```python
from build123d import *

# Parameters (mm, degrees)
F0_W     = 239.2428293824
F0_H     = 256.9792084396
F2_DEPTH = 82.55
F3_T     = -2
F4_DEPTH = 2


with BuildPart() as f2:
    # F0 (on Top) → F2 (new body)
    with BuildSketch(Plane.XY):
        with Locations((-25.7889069617, 128.4896042198)):
            Rectangle(F0_W, F0_H)
    extrude(amount=F2_DEPTH)

    # F3
    f3_openings = [f2.faces().sort_by_distance(p)[0] for p in [
        (-25.788907, 128.489604, 82.55),
    ]]
    offset(amount=F3_T, openings=f3_openings)

    # F0 (on Top) → F4 (join)
    with BuildSketch(Plane.XY):
        with Locations((-25.7889069617, 128.4896042198)):
            Rectangle(F0_W, F0_H)
    extrude(amount=F4_DEPTH)


solid = f2.part
```
The model under review builds one solid part; all positions refer to its coordinate system, in mm. A direction names the side the tool comes from. Give positions to 0.01 mm unless a question says otherwise; leave off trailing zeros. Write each loop counter-clockwise with the first axis right and the second up, starting at its lowest first coordinate (ties: lowest second). Pieces come first, ordered by that corner, then holes. Notation, with made-up numbers: (9, 65.25) - (59, 65.25) arc R18 cw to (59, 72.25) - close; hole circle Ø11 at (39.5, 13.25). An arc over 180 degrees is marked (long way). Answer in a Markdown table with one row per item. Add a question column.
1. Wall thickness on line 1 along X through (y, z) = (54.5, 62); line 2 along Y through (x, z) = (-51, 50.5); line 3 along Z through (x, y) = (24.5, 92): over which ranges is each line inside the solid? List them lowest first. Write a range as [from, to].
2. We need section A-A on z = 43. Write out the cut boundary in (x, y).
3. Insertion check: P1, Ø4, axis at x = 58.5, y = 217.5, coming from the +Z side. The pin has a flat end and moves straight along its axis. Give the tip position at first contact, or say it passes through.
4. Tool access review of faces 1 (the flat face through (-27, 130, 2)), 2 (the flat face through (93.833, 127, 41)): name each direction out of +Z, -Z, +X, -X, +Y, -Y from which nothing blocks a thin tool from reaching the whole face with its end or side.
5. Draft analysis for pull direction Y (two halves, no side actions). For faces 3 (the flat face through (-145.41, 127, 41)), 4 (the flat face through (-27, 256.979, 41)), 5 (the flat face through (91.833, 127, 42)), 6 (the flat face through (-27, 254.979, 42)), state which applies: +Y half, -Y half, draft (parallel to the pull), parting line (faces both ways), or undercut.
6. We need section C-C on x = 48. Write out the cut boundary in (y, z), then the cut area to 3 significant figures.
7. We need section B-B on y = 103. Write out the cut boundary in (x, z).
Ans:
| question | item | result |
|---|---|---|
| 1 | line 1 | x = [-145.41, -143.41], [91.83, 93.83] |
| 1 | line 2 | y = [0, 2], [254.98, 256.98] |
| 1 | line 3 | z = [0, 2] |
| 2 | outline | (-145.41, 0) - (93.83, 0) - (93.83, 256.98) - (-145.41, 256.98) - close; hole (-143.41, 2) - (91.83, 2) - (91.83, 254.98) - (-143.41, 254.98) - close |
| 3 | P1 | stops at z = 2 |
| 4 | face 1 | +Z |
| 4 | face 2 | +Z, -Z, +X, +Y, -Y |
| 5 | face 3 | draft |
| 5 | face 4 | +Y half |
| 5 | face 5 | undercut |
| 5 | face 6 | undercut |
| 6 | outline | (0, 0) - (256.98, 0) - (256.98, 82.55) - (254.98, 82.55) - (254.98, 2) - (2, 2) - (2, 82.55) - (0, 82.55) - close |
| 6 | area | 836 mm^2 |
| 7 | outline | (-145.41, 0) - (93.83, 0) - (93.83, 82.55) - (91.83, 82.55) - (91.83, 2) - (-143.41, 2) - (-143.41, 82.55) - (-145.41, 82.55) - close |
